Design review of the part built by this model. Coordinates are the model's own, in mm. A direction names the side the tool comes from. Coordinates: 2 decimals unless noted, no trailing zeros. Loops run counter-clockwise (first coordinate to the right, second up) from the corner with the lowest first, then second, coordinate; pieces in that order, holes last. Notation, with made-up numbers: (45, 23) -> (74, 23) arc R15 cw to (74, 50) -> close; hole circle Ø7 at (35.25, -21). An arc over 180 degrees is marked (long way). One line per item, written item: value. Start each with the question number.
1. Insertion check: pin 1 (2.5 mm diameter, centred on x = -5.5, y = -12.5, fed in from +Z) (3 decimals); pin 2 (0.9 mm diameter, centred on y = -15, z = 19, fed in from -X); pin 3 (5.5 mm diameter, centred on x = 101.5, z = 19, fed in from +Y); pin 4 (1 mm diameter, centred on y = -10.5, z = 16.5, fed in from -X). Each pin has a flat end and moves straight along its axis. Give the tip position at first contact, or say it passes through.
2. Add section A-A on z = 15. Give the number of separate pieces and of enclosed holes in the cut face, plus the area to 3 significant figures.
3. Draft analysis for pull direction X (two halves, no side actions). For faces 1 (the flat face through (-10, -12, 34)), 2 (the cylindrical face through (98.29, -11.01, 19.72)), 3 (the flat face through (101, -10, 20)), 4 (the cylindrical face through (104.695, -11.177, 19.72)), state which applies: pulls with the +X half, pulls with the -X half, needs draft (parallel to the pull), parting line crosses it, or undercut.
4. For probe 1 along Y at (x, z) = (-5.5, 34); probe 2 along X at (y, z) = (-12.5, 8.75) (3 decimals); probe 3 along Z at (x, y) = (32.5, -14.5), list the stretches that pass through material, from the lowest coordinate up.
5. Add section D-D on x = 0. Write out the cut boundary in (y, z), plus the area to 3 significant figures.
6. Machinability: for faces 5 (the flat face through (77.78, -15.52, 18.47)), 6 (the flat face through (-10, -12, 6)), 7 (the cylindrical face through (97.3, -13.5, 19.7)), which of the approach directions +Z, -Z, +X, -X, +Y, -Y give a long, thin tool a straight path to every point of the face, cutting with its end or side? Answer none if there is none.
7. Add section C-C on z = 35.5. Write out the cut boundary in (x, y) (3 decimals), plus the area to 3 significant figures.
8. Add section B-B on x = 80. Write out the cut boundary in (y, z).
Autodesk Inventor part; units mm, degrees
ref_plane "Płaszczyzna konstrukcyjna1" through (101.455, -9, 0) normal (0, 1, 0) x (-1, 0, 0)
ref_plane "YZ Plane" through (0, 0, 0) normal (1, 0, 0) x (0, 1, 0)
ref_plane "XZ Plane" through (0, 0, 0) normal (0, 1, 0) x (-1, 0, 0)
sketch "Szkic1" plane through (0, 0, 0) normal (0, 0, 1) x (1, 0, 0)
  circle A0 centre (-5.5, -12.5) radius 1.5
  circle A1 centre (-5.5, 53.1646) radius 1.5
  circle A2 centre (101.455, -12.5) radius 1.5
  arc A3 (-10, -15) -> (-8, -17) centre (-8, -15) ccw
  line L0 (-8, -17) -> (136.455, -17)
  arc A4 (136.455, -17) -> (141.455, -12) centre (136.455, -12) ccw
  line L1 (141.455, -12) -> (141.455, -2)
  arc A5 (141.455, -2) -> (136.455, 3) centre (136.455, -2) ccw
  line L2 (136.455, 3) -> (127.455, 3)
  arc A6 (115.455, 15) -> (127.455, 3) centre (127.455, 15) ccw
  line L3 (115.455, 15) -> (115.455, 29.1646)
  arc A7 (127.455, 41.1646) -> (115.455, 29.1646) centre (127.455, 29.1646) ccw
  line L4 (127.455, 41.1646) -> (136.455, 41.1646)
  arc A8 (136.455, 41.1646) -> (141.455, 46.1646) centre (136.455, 46.1646) ccw
  line L5 (141.455, 46.1646) -> (141.455, 56.1646)
  arc A9 (141.455, 56.1646) -> (136.455, 61.1646) centre (136.455, 56.1646) ccw
  line L6 (136.455, 61.1646) -> (122.455, 61.1646)
  line L7 (107.455, 76.1646) -> (122.455, 61.1646)
  line L8 (107.455, 76.1646) -> (107.455, 88.1646)
  arc A10 (107.455, 88.1646) -> (102.455, 93.1646) centre (102.455, 88.1646) ccw
  line L9 (102.455, 93.1646) -> (92.455, 93.1646)
  arc A11 (92.455, 93.1646) -> (87.455, 88.1646) centre (92.455, 88.1646) ccw
  line L10 (87.455, 88.1646) -> (87.455, 79.1646)
  arc A12 (75.455, 67.1646) -> (87.455, 79.1646) centre (75.455, 79.1646) ccw
  line L11 (75.455, 67.1646) -> (22, 67.1646)
  arc A13 (10, 79.1646) -> (22, 67.1646) centre (22, 79.1646) ccw
  line L12 (10, 79.1646) -> (10, 88.1646)
  arc A14 (10, 88.1646) -> (5, 93.1646) centre (5, 88.1646) ccw
  line L13 (5, 93.1646) -> (-5, 93.1646)
  arc A15 (-5, 93.1646) -> (-10, 88.1646) centre (-5, 88.1646) ccw
  line L14 (-10, 88.1646) -> (-10, -15)
  circle A16 centre (97.455, 83.1646) radius 2
  circle A17 centre (131.455, -7) radius 2
  circle A18 centre (131.455, 51.1646) radius 2
  circle A19 centre (0, 83.1646) radius 2
  line L15 (89.5711, 35.5361) -> (89.5711, 17.5361)
  arc A20 (83.5711, 11.5361) -> (89.5711, 17.5361) centre (83.5711, 17.5361) ccw
  line L16 (83.5711, 11.5361) -> (78.5711, 11.5361)
  arc A21 (72.5711, 17.5361) -> (78.5711, 11.5361) centre (78.5711, 17.5361) ccw
  line L17 (72.5711, 17.5361) -> (72.5711, 35.5361)
  arc A22 (78.5711, 41.5361) -> (72.5711, 35.5361) centre (78.5711, 35.5361) ccw
  line L18 (78.5711, 41.5361) -> (83.5711, 41.5361)
  arc A23 (89.5711, 35.5361) -> (83.5711, 41.5361) centre (83.5711, 35.5361) ccw
  line L19 (107.455, 22.1646) -> (107.455, 25.6646)
  line L20 (107.455, 25.6646) -> (109.455, 25.6646)
  line L21 (109.455, 25.6646) -> (109.455, 22.1646)
  line L22 (109.455, 22.1646) -> (107.455, 22.1646)
  line L23 (82.5, 60.1646) -> (86, 60.1646)
  line L24 (86, 60.1646) -> (86, 58.1646)
  line L25 (86, 58.1646) -> (82.5, 58.1646)
  line L26 (82.5, 58.1646) -> (82.5, 60.1646)
  line L27 (53.5, 60.1646) -> (57, 60.1646)
  line L28 (57, 60.1646) -> (57, 58.1646)
  line L29 (57, 58.1646) -> (53.5, 58.1646)
  line L30 (53.5, 58.1646) -> (53.5, 60.1646)
  line L31 (24.5, 60.1646) -> (28, 60.1646)
  line L32 (28, 60.1646) -> (28, 58.1646)
  line L33 (28, 58.1646) -> (24.5, 58.1646)
  line L34 (24.5, 58.1646) -> (24.5, 60.1646)
  line L35 (10, 58.1646) -> (10, 60.1646)
  line L36 (10, 60.1646) -> (13.5, 60.1646)
  line L37 (13.5, 60.1646) -> (13.5, 58.1646)
  line L38 (13.5, 58.1646) -> (10, 58.1646)
  line L39 (39, 60.1646) -> (42.5, 60.1646)
  line L40 (42.5, 60.1646) -> (42.5, 58.1646)
  line L41 (42.5, 58.1646) -> (39, 58.1646)
  line L42 (39, 58.1646) -> (39, 60.1646)
  line L43 (68, 60.1646) -> (71.5, 60.1646)
  line L44 (71.5, 60.1646) -> (71.5, 58.1646)
  line L45 (71.5, 58.1646) -> (68, 58.1646)
  line L46 (68, 58.1646) -> (68, 60.1646)
  line L47 (107.455, 37.6646) -> (107.455, 41.1646)
  line L48 (107.455, 41.1646) -> (109.455, 41.1646)
  line L49 (109.455, 41.1646) -> (109.455, 37.6646)
  line L50 (109.455, 37.6646) -> (107.455, 37.6646)
  line L51 (107.455, 6.6646) -> (107.455, 10.1646)
  line L52 (107.455, 10.1646) -> (109.455, 10.1646)
  line L53 (109.455, 10.1646) -> (109.455, 6.6646)
  line L54 (109.455, 6.6646) -> (107.455, 6.6646)
  line L55 (54.7961, 40.5361) -> (54.7961, 12.5361)
  arc A24 (48.7961, 6.5361) -> (54.7961, 12.5361) centre (48.7961, 12.5361) ccw
  line L56 (48.7961, 6.5361) -> (30.7961, 6.5361)
  arc A25 (24.7961, 12.5361) -> (30.7961, 6.5361) centre (30.7961, 12.5361) ccw
  line L57 (24.7961, 12.5361) -> (24.7961, 40.5361)
  arc A26 (30.7961, 46.5361) -> (24.7961, 40.5361) centre (30.7961, 40.5361) ccw
  line L58 (30.7961, 46.5361) -> (48.7961, 46.5361)
  arc A27 (54.7961, 40.5361) -> (48.7961, 46.5361) centre (48.7961, 40.5361) ccw
  circle A28 centre (65.8311, 7.4861) radius 1.6
  circle A29 centre (15.0311, 50.6661) radius 1.6
  circle A30 centre (89.9611, 50.6661) radius 1.6
  circle A31 centre (13.7611, 2.4061) radius 1.6
  circle A32 centre (65.8311, 35.4261) radius 1.6
  circle A33 centre (96.3111, 2.4061) radius 1.6
  line L59 (105.455, -17) -> (105.455, -14)
  line L60 (105.455, -14) -> (-10, -14)
  arc A34 (-2.3377, -14) -> (-8.6623, -14) centre (-5.5, -12.5) ccw
  arc A35 (104.6173, -14) -> (98.2927, -14) centre (101.455, -12.5) ccw
  line L61 (-5.5, -9) -> (-10, -9)
  point P0 (0, 0)
  point P1 (0, 0)
  dimension "d0" = 3
  dimension "d1" = 36
  dimension "d2" = 7
  dimension "d3" = 7
extrude "Wyciągnięcie proste1" add sketch "Szkic1" along normal blind 40 contours L60 A34 | L60 L59 L0 A3 L14 | L60 L14 L61 A34 | A35 L60
fillet "Zaokrąglenie1" radius 2 2 edges at (98.2927, -14, 20) (104.6173, -14, 20)
fillet "Zaokrąglenie1" radius 0.8 1 edges at (-2.3377, -14, 20)
sketch "Szkic2" plane through (-8, -17, 0) normal (0, -1, 0) x (1, 0, 0)
  line L0 (0, 0) -> (113.455, 0)
  line L1 (113.455, 0) -> (113.455, 40)
  line L2 (0, 40) -> (113.455, 40)
  line L3 (0, 0) -> (0, 40)
  line L4 (-2, 0) -> (-2, 40)
  line L5 (-2, 0) -> (-2, 40)
  line L6 (-2, 27.75) -> (6.5, 27.75)
  line L7 (6.5, 27.75) -> (6.5, 12.25)
  line L8 (6.5, 12.25) -> (-2, 12.25)
  line L9 (-2, 12.25) -> (-2, 27.75)
  point P0 (8, 0)
  dimension "d7" = 8.5
  dimension "d8" = 15.5
  dimension "d9" = 40
  dimension "d10" = 12.25
extrude "Wyciągnięcie proste2" cut sketch "Szkic2" against normal through all contours L8 L4 L6 L3 | L3 L6 L7 L8
sketch "Szkic3" plane through (-8, -17, 0) normal (0, -1, 0) x (1, 0, 0)
  line L0 (6.5, 12.25) -> (0, 12.25)
  line L1 (0, 0) -> (0, 12.25)
  line L2 (0, 0) -> (113.455, 0)
  line L3 (113.455, 0) -> (113.455, 40)
  line L4 (0, 40) -> (113.455, 40)
  line L5 (0, 27.75) -> (0, 40)
  line L6 (0, 27.75) -> (6.5, 27.75)
  line L7 (6.5, 27.75) -> (6.5, 12.25)
  line L8 (103.9778, 0) -> (103.9778, 40)
  line L9 (17.5103, 11.5147) -> (34.4808, 28.4853) construction
  line L10 (18.9245, 10.1005) -> (35.8951, 27.0711)
  line L11 (33.0666, 29.8995) -> (16.0961, 12.9289)
  arc A0 (16.0961, 12.9289) -> (18.9245, 10.1005) centre (17.5103, 11.5147) ccw
  arc A1 (35.8951, 27.0711) -> (33.0666, 29.8995) centre (34.4808, 28.4853) ccw
  line L12 (25.9956, 20) -> (49.9956, 20) construction
  line L13 (37.0058, 11.5147) -> (53.9764, 28.4853) construction
  line L14 (38.42, 10.1005) -> (55.3906, 27.0711)
  line L15 (52.5622, 29.8995) -> (35.5916, 12.9289)
  arc A2 (35.5916, 12.9289) -> (38.42, 10.1005) centre (37.0058, 11.5147) ccw
  arc A3 (55.3906, 27.0711) -> (52.5622, 29.8995) centre (53.9764, 28.4853) ccw
  line L16 (45.4911, 20) -> (69.4911, 20) construction
  line L17 (56.5014, 11.5147) -> (73.472, 28.4853) construction
  line L18 (57.9156, 10.1005) -> (74.8862, 27.0711)
  line L19 (72.0577, 29.8995) -> (55.0872, 12.9289)
  arc A4 (55.0872, 12.9289) -> (57.9156, 10.1005) centre (56.5014, 11.5147) ccw
  arc A5 (74.8862, 27.0711) -> (72.0577, 29.8995) centre (73.472, 28.4853) ccw
  line L20 (64.9867, 20) -> (88.9867, 20) construction
  line L21 (75.997, 11.5147) -> (92.9675, 28.4853) construction
  line L22 (77.4112, 10.1005) -> (94.3817, 27.0711)
  line L23 (91.5533, 29.8995) -> (74.5827, 12.9289)
  arc A6 (74.5827, 12.9289) -> (77.4112, 10.1005) centre (75.997, 11.5147) ccw
  arc A7 (94.3817, 27.0711) -> (91.5533, 29.8995) centre (92.9675, 28.4853) ccw
  line L24 (84.4822, 20) -> (108.4822, 20) construction
  arc A8 (45.8917, 23.229) -> (41.926, 19.2633) centre (43.155, 22) ccw
  point P0 (8, 0)
  dimension "d13" = 40
  dimension "d14" = 20
  dimension "d15" = 20
  dimension "d16" = 20
  dimension "d17" = 20
  dimension "d19" = 97.4778
  dimension "d20" = 19.4956
  dimension "d21" = 19.4956
  dimension "d22" = 19.4956
  dimension "d23" = 19.4956
  dimension "d24" = 12
  dimension "d25" = 45
  dimension "d26" = 4
  dimension "d27" = 12
  dimension "d28" = 45
  dimension "d29" = 4
  dimension "d30" = 12
  dimension "d31" = 45
  dimension "d32" = 4
  dimension "d33" = 12
  dimension "d34" = 45
  dimension "d35" = 4
  dimension "d38" = 18
  dimension "d39" = 70.3
  dimension "d40" = 6
extrude "Wyciągnięcie proste3" cut sketch "Szkic3" against normal through all contours A0 L11 A1 L10 | A2 L15 A3 L14 | A8 L15 | A4 L19 A5 L18 | A6 L23 A7 L22
fillet "Zaokrąglenie2" radius 2 2 edges at (33.926, -15.5, 19.2633) (37.8917, -15.5, 23.229)
ref_plane "Płaszczyzna konstrukcyjna1" through (101.455, -9, 0) normal (0, 1, 0) x (-1, 0, 0)
sketch "Szkic4" plane through (101.455, -9, 0) normal (0, 1, 0) x (-1, 0, 0)
  line L0 (16.8478, 48.5064) -> (-17.7331, 48.5064)
  line L1 (-17.7331, 48.5064) -> (-17.7331, -24.0755)
  line L2 (-17.7331, -24.0755) -> (16.8478, -24.0755)
  line L3 (16.8478, -24.0755) -> (16.8478, 48.5064)
  point P0 (101.455, 0)
extrude "Wyciągnięcie proste4" cut sketch "Szkic4" against normal blind 1
equation "\"d10\" = -0.5 * d8 + 0.5 * d9"
equation "\"d16\" = d15"
equation "\"d17\" = d15"
equation "\"d20\" = 0.2 * d19"
equation "\"d21\" = d20"
equation "\"d22\" = d20"
equation "\"d23\" = d20"
properties part number "3DP_PLA_Controller_Case_Side_Wall_Longer"
Worked answers:
1. pin 1: passes through
1. pin 2: stops at x = -1.5
1. pin 3: stops at y = -10
1. pin 4: stops at x = 98.29
2. separate pieces: 5
2. enclosed holes: 1
2. area: 273 mm²
3. face 1: pulls with the -X half
3. face 2: undercut
3. face 3: needs draft
3. face 4: pulls with the +X half
4. probe 1: y = -17 to -14, -11 to -9
4. probe 2: x = -10 to -7, -4 to -2, 97.914 to 99.955, 102.955 to 104.955
4. probe 3: z = 0 to 12.18, 17.84 to 20.6, 23.4 to 40
5. outline: (-17, 0) -> (-14, 0) -> (-14, 40) -> (-17, 40) -> close
5. area: 120 mm²
6. face 5: +Y, -Y
6. face 6: +Z, -Z, -X, +Y, -Y
6. face 7: +Z, -Z, +Y
7. outline: (-10, -15) arc R2 ccw to (-8, -17) -> (105.455, -17) -> (105.455, -14) arc R2 cw to (104.953, -12.611) arc R3.5 ccw to (103.905, -10) -> (99.005, -10) arc R3.5 ccw to (97.969, -12.182) arc R2 cw to (95.978, -14) -> (-1.257, -14) arc R0.8 cw to (-2.047, -13.07) arc R3.5 ccw to (-5.5, -9) -> (-10, -9) -> close; hole circle Ø3 at (-5.5, -12.5); hole circle Ø3 at (101.455, -12.5)
7. area: 396 mm²
8. outline: (-17, 0) -> (-14, 0) -> (-14, 20.69) -> (-17, 20.69) -> close; (-17, 26.35) -> (-14, 26.35) -> (-14, 40) -> (-17, 40) -> close
